Input: part model. Units: mm. Frame: model coordinates. A direction names the side the tool comes from. Coordinates: 2 decimals unless noted, no trailing zeros. Order: outer loops, then holes, each group sorted by start corner. A loop starts at its lowest first (then second) coordinate and runs counter-clockwise, first axis right, second up. Notation, with made-up numbers: (38.5, 5) -> (59.5, 5) arc R18 cw to (59.5, 26) -> close; hole circle Ø8 at (64, 70). An arc over 180 degrees is marked (long way). Answer as CSV lines item,"result".
from build123d import *

# Parameters (mm, degrees)
BOSS_EXTRUDE1_DEPTH = 90
CUT_EXTRUDE2_DEPTH  = 100
CIRPATTERN3_COUNT   = 6


with BuildPart() as part:
    # Sketch1 → Boss-Extrude1 (new body)
    with BuildSketch(Plane.XY):
        with BuildLine():
            Line((-14.058688457, 5.230036219), (-40.22114317, 20.334936491))
            Line((-40.22114317, 20.334936491), (-37.72114317, 24.665063509))
            Line((-37.72114317, 24.665063509), (-11.558688457, 9.560163238))
            ThreePointArc((-11.558688457, 9.560163238), (-9.682458366, 11.456439237), (-7.5, 12.990381057))
            Line((-7.5, 12.990381057), (0, 0))
            Line((0, 0), (-15, 0))
            ThreePointArc((-15, 0), (-14.762796599, 2.657035297), (-14.058688457, 5.230036219))
        make_face()
    boss_extrude1 = extrude(amount=BOSS_EXTRUDE1_DEPTH)

    # Sketch2 → Cut-Extrude2 (cut)
    with BuildSketch(Plane(origin=(1.25, 2.165063509, 0), x_dir=(0.8660254037844417, -0.4999999999999949, 0), z_dir=(0.4999999999999949, 0.8660254037844417, 0))):
        with BuildLine():
            Line((-45, 0), (-45, -45))
            ThreePointArc((-45, -45), (-36.747126088, -17.900036675), (-14.790199458, 0))
            Line((-14.790199458, 0), (-45, 0))
        make_face()
        with BuildLine():
            Line((-45, -90), (-14.790199458, -90))
            ThreePointArc((-14.790199458, -90), (-36.747126088, -72.099963325), (-45, -45))
            Line((-45, -45), (-45, -90))
        make_face()
    cut_extrude2 = extrude(amount=-CUT_EXTRUDE2_DEPTH, mode=Mode.SUBTRACT)

    # CirPattern3: Boss-Extrude1, Cut-Extrude2 ×6 about axis
    cirpattern3_axis = Axis((0, 0, 0), (0, 0, 1))
    add([boss_extrude1.rotate(cirpattern3_axis, i * 360 / CIRPATTERN3_COUNT) for i in range(1, CIRPATTERN3_COUNT)])
    add([cut_extrude2.rotate(cirpattern3_axis, i * 360 / CIRPATTERN3_COUNT) for i in range(1, CIRPATTERN3_COUNT)], mode=Mode.SUBTRACT)


solid = part.part
1. Mould query, pull axis Y, two halves, no side actions, for faces 1 (the face through (-21.5, -15.3, 44.4)), 2 (the face through (-24.05, 11, 44.37)), 3 (the face through (0, 0, 90)), 4 (the face through (-21.92, 15.54, 44.37)). Classes: released by +Y, released by -Y, zero draft, split by the parting line, or undercut.
Findings:
face 1,"released by -Y"
face 2,"undercut"
face 3,"zero draft"
face 4,"released by +Y"
2. Cut plane A-A (z = 58). Return the cut outline in (x, y).
Findings:
outline,"(-38.69, -19.45) -> (-36.19, -23.78) -> (-11.56, -9.56) arc R15 ccw to (-2.5, -14.79) -> (-2.5, -43.23) -> (2.5, -43.23) -> (2.5, -14.79) arc R15 ccw to (11.56, -9.56) -> (36.19, -23.78) -> (38.69, -19.45) -> (14.06, -5.23) arc R15 ccw to (14.06, 5.23) -> (38.69, 19.45) -> (36.19, 23.78) -> (11.56, 9.56) arc R15 ccw to (2.5, 14.79) -> (2.5, 43.23) -> (-2.5, 43.23) -> (-2.5, 14.79) arc R15 ccw to (-11.56, 9.56) -> (-36.19, 23.78) -> (-38.69, 19.45) -> (-14.06, 5.23) arc R15 ccw to (-14.06, -5.23) -> close"
3. Cut plane B-B (y = -16). State how many separate pieces and enclosed holes the cut face has, plus the area to 3 significant figures.
Findings:
separate pieces,"3"
enclosed holes,"0"
area,"1,760 mm2"
4. Cut plane C-C (y = 33.5). Return the cut outline in (x, z).
Findings:
outline,"(-2.5, 13.6) -> (2.5, 13.6) -> (2.5, 76.4) -> (-2.5, 76.4) -> close"
5. Ray query, line 1 along X through (y, z) = (-11.5, 86); line 2 along X through (y, z) = (-18, 25.5); line 3 along X through (y, z) = (24.5, 33). Return the intervals inside material, ascending.
Findings:
line 1,"x = -19.36 to -14.92, -9.63 to 9.63, 14.92 to 19.36"
line 2,"x = -36.18 to -26.18, -2.5 to 2.5, 26.18 to 36.18"
line 3,"x = -2.5 to 2.5"
6. Cut plane D-D (z = 11.5). Return the cut outline in (x, y), plus the area to 3 significant figures.
Findings:
outline,"(-28.63, -13.64) -> (-26.13, -17.97) -> (-11.56, -9.56) arc R15 ccw to (-2.5, -14.79) -> (-2.5, -31.62) -> (2.5, -31.62) -> (2.5, -14.79) arc R15 ccw to (11.56, -9.56) -> (26.13, -17.97) -> (28.63, -13.64) -> (14.06, -5.23) arc R15 ccw to (14.06, 5.23) -> (28.63, 13.64) -> (26.13, 17.97) -> (11.56, 9.56) arc R15 ccw to (2.5, 14.79) -> (2.5, 31.62) -> (-2.5, 31.62) -> (-2.5, 14.79) arc R15 ccw to (-11.56, 9.56) -> (-26.13, 17.97) -> (-28.63, 13.64) -> (-14.06, 5.23) arc R15 ccw to (-14.06, -5.23) -> close"
area,"1,210 mm2"
7. Contact query for flat-ended pins moving along their axis: pin 1 (6 mm diameter, centred on y = -31, z = 25, fed in from +X); pin 2 (10 mm diameter, centred on y = -11, z = 19, fed in from -X); pin 3 (1.5 mm diameter, centred on x = -0.5, y = 32.5, fed in from -Z). Output: stop coordinate, or through.
Findings:
pin 1,"stops at x = 2.5"
pin 2,"stops at x = -32.71"
pin 3,"stops at z = 11.64"
8. Reachability of faces 5 (the face through (-2.5, 26, 44)), 6 (the face through (-24.4, -11.2, 44.4)), 7 (the face through (24.4, 11.2, 44.4)) from +Z, -Z, +X, -X, +Y, -Y: full face, straight path, thin tool, end or side. Return the list, or none.
Findings:
face 5,"+Z, -Z, +Y"
face 6,"+Z, -Z, -X"
face 7,"+Z, -Z, +X"
